```python
from build123d import *

# Parameters (mm, degrees)
SKETCH_1_R          = 103
EXTRUDE_1_DEPTH     = 3
SKETCH_2_W          = 30
SKETCH_2_H          = 42
SKETCH_2_W_2        = 24
SKETCH_2_H_2        = 32
EXTRUDE_2_DEPTH     = 25
SKETCH_3_R          = 0.5
CUT_EXTRUDE_1_DEPTH = 25
CUT_EXTRUDE_2_DEPTH = 25
SKETCH_5_R          = 103
SKETCH_5_R_2        = 100.319489632
EXTRUDE_3_DEPTH     = 50
SKETCH_6_W          = 139.713993572
SKETCH_6_H          = 16
SKETCH_6_W_2        = 184
SKETCH_6_W_3        = 75
CUT_EXTRUDE_3_DEPTH = 50
EXTRUDE_START       = -5
SKETCH_7_R          = 103
SKETCH_7_R_2        = 98
EXTRUDE_4_DEPTH     = 5
SKETCH_8_R          = 100
SKETCH_8_R_2        = 98
EXTRUDE_5_DEPTH     = 5
EXTRUDE_6_DEPTH     = 25
SKETCH_10_W         = 24
SKETCH_10_H         = 32
SKETCH_10_W_2       = 12.5
SKETCH_10_H_2       = 24
EXTRUDE_7_DEPTH     = 25
SKETCH_11_R         = 25.806975801
SKETCH_11_W         = 12.5
SKETCH_11_H         = 24
CUT_EXTRUDE_4_DEPTH = 8
SKETCH_12_W         = 12.5
SKETCH_12_H         = 24
CUT_EXTRUDE_5_DEPTH = 8
SKETCH_13_W         = 12.5
SKETCH_13_H         = 5.2
CUT_EXTRUDE_6_DEPTH = 100
SKETCH_14_R         = 103
SKETCH_14_R_2       = 98
EXTRUDE_9_DEPTH     = 50
SKETCH_15_W         = 3
SKETCH_15_H         = 9
CUT_EXTRUDE_7_DEPTH = 70


with BuildPart() as part:
    # 草图1 → 凸台-拉伸1 (new body)
    with BuildSketch(Plane(origin=(0, 0, 0), x_dir=(1, 0, 0), z_dir=(0, 1, 0))):
        with Locations(Location((0, 0, 0), (0, 0, 270))):
            Circle(SKETCH_1_R)
    extrude(amount=EXTRUDE_1_DEPTH)

    # 草图2 → 凸台-拉伸2 (add)
    with BuildSketch(Plane(origin=(0, 3, 0), x_dir=(1, 0, 0), z_dir=(0, 1, 0))):
        Rectangle(SKETCH_2_W, SKETCH_2_H)
        Rectangle(SKETCH_2_W_2, SKETCH_2_H_2, mode=Mode.SUBTRACT)
    extrude(amount=EXTRUDE_2_DEPTH)

    # 草图3 → 切除-拉伸1 (cut)
    with BuildSketch(Plane(origin=(0, 28, 0), x_dir=(1, 0, 0), z_dir=(0, 1, 0))):
        with Locations(Location((0, -18.5, 0), (0, 0, 270))):
            Circle(SKETCH_3_R)
        with Locations(Location((0, 18.5, 0), (0, 0, 270))):
            Circle(SKETCH_3_R)
    extrude(amount=-CUT_EXTRUDE_1_DEPTH, mode=Mode.SUBTRACT)

    # 草图4 → 切除-拉伸2 (cut)
    with BuildSketch(Plane(origin=(0, 3, 0), x_dir=(1, 0, 0), z_dir=(0, 1, 0))):
        Polygon((25, 0), (25, -8), (100, -8), (100, 0), (100, 8), (25, 8), align=None)
    extrude(amount=-CUT_EXTRUDE_2_DEPTH, mode=Mode.SUBTRACT)

    # 草图5 → 凸台-拉伸3 (add)
    with BuildSketch(Plane(origin=(0, 3, 0), x_dir=(1, 0, 0), z_dir=(0, 1, 0))):
        with Locations(Location((0, 0, 0), (0, 0, 270))):
            Circle(SKETCH_5_R)
        with Locations(Location((0, 0, 0), (0, 0, 4.57392126))):
            Circle(SKETCH_5_R_2, mode=Mode.SUBTRACT)
    extrude(amount=EXTRUDE_3_DEPTH)

    # 草图6 → 切除-拉伸3 (cut)
    with BuildSketch(Plane(origin=(0, 3, 0), x_dir=(1, 0, 0), z_dir=(0, 1, 0))):
        with Locations((0, -64)):
            Rectangle(SKETCH_6_W, SKETCH_6_H)
        with Locations((0, -32)):
            Rectangle(SKETCH_6_W_2, SKETCH_6_H)
        with Locations((-62.5, 0)):
            Rectangle(SKETCH_6_W_3, SKETCH_6_H)
        with Locations((0, 32)):
            Rectangle(SKETCH_6_W_2, SKETCH_6_H)
        with Locations((0, 64)):
            Rectangle(SKETCH_6_W, SKETCH_6_H)
    extrude(amount=-CUT_EXTRUDE_3_DEPTH, mode=Mode.SUBTRACT)

    # 草图7 → 凸台-拉伸4 (add)
    with BuildSketch(Plane(origin=(0, 53, 0), x_dir=(1, 0, 0), z_dir=(0, 1, 0)).offset(EXTRUDE_START)):
        with Locations(Location((0, 0, 0), (0, 0, 270))):
            Circle(SKETCH_7_R)
        with Locations(Location((0, 0, 0), (0, 0, 270))):
            Circle(SKETCH_7_R_2, mode=Mode.SUBTRACT)
    extrude(amount=EXTRUDE_4_DEPTH)

    # 草图8 → 凸台-拉伸5 (add)
    with BuildSketch(Plane(origin=(0, 53, 0), x_dir=(1, 0, 0), z_dir=(0, 1, 0))):
        with Locations(Location((0, 0, 0), (0, 0, 270))):
            Circle(SKETCH_8_R)
        with Locations(Location((0, 0, 0), (0, 0, 270))):
            Circle(SKETCH_8_R_2, mode=Mode.SUBTRACT)
    extrude(amount=EXTRUDE_5_DEPTH)

    # 草图9 → 凸台-拉伸6 (add)
    with BuildSketch(Plane(origin=(0, 28, 0), x_dir=(1, 0, 0), z_dir=(0, 1, 0))):
        with BuildLine():
            ThreePointArc((25.806975801, 0), (22.946727839, 11.808796784), (15, 21))
            Line((15, 21), (15, -21))
            ThreePointArc((15, -21), (22.946727839, -11.808796784), (25.806975801, 0))
        make_face()
        with BuildLine():
            ThreePointArc((15, 21), (0, 25.806975801), (-15, 21))
            Line((-15, 21), (15, 21))
        make_face()
        with BuildLine():
            Line((-15, -21), (-15, 21))
            ThreePointArc((-15, 21), (-25.806975801, 0), (-15, -21))
        make_face()
        with BuildLine():
            Line((15, -21), (-15, -21))
            ThreePointArc((-15, -21), (0, -25.806975801), (15, -21))
        make_face()
    extrude(amount=-EXTRUDE_6_DEPTH)

    # 草图10 → 凸台-拉伸7 (add)
    with BuildSketch(Plane(origin=(0, 28, 0), x_dir=(1, 0, 0), z_dir=(0, 1, 0))):
        Rectangle(SKETCH_10_W, SKETCH_10_H)
        Rectangle(SKETCH_10_W_2, SKETCH_10_H_2, mode=Mode.SUBTRACT)
    extrude(amount=-EXTRUDE_7_DEPTH)

    # 草图11 → 切除-拉伸4 (cut)
    with BuildSketch(Plane(origin=(0, 28, 0), x_dir=(1, 0, 0), z_dir=(0, 1, 0))):
        with Locations(Location((0, 0, 0), (0, 0, 270))):
            Circle(SKETCH_11_R)
        Rectangle(SKETCH_11_W, SKETCH_11_H, mode=Mode.SUBTRACT)
    extrude(amount=-CUT_EXTRUDE_4_DEPTH, mode=Mode.SUBTRACT)

    # 草图12 → 切除-拉伸5 (cut)
    with BuildSketch(Plane.XZ):
        Rectangle(SKETCH_12_W, SKETCH_12_H)
    extrude(amount=-CUT_EXTRUDE_5_DEPTH, mode=Mode.SUBTRACT)

    # 草图13 → 切除-拉伸6 (cut)
    with BuildSketch(Plane(origin=(0, 20, 0), x_dir=(1, 0, 0), z_dir=(0, 1, 0))):
        with Locations((0, -14.6)):
            Rectangle(SKETCH_13_W, SKETCH_13_H)
    extrude(amount=-CUT_EXTRUDE_6_DEPTH, mode=Mode.SUBTRACT)

    # 草图14 → 凸台-拉伸9 (add)
    with BuildSketch(Plane(origin=(0, 3, 0), x_dir=(1, 0, 0), z_dir=(0, 1, 0))):
        with Locations(Location((0, 0, 0), (0, 0, 270))):
            Circle(SKETCH_14_R)
        with Locations(Location((0, 0, 0), (0, 0, 270))):
            Circle(SKETCH_14_R_2, mode=Mode.SUBTRACT)
    extrude(amount=EXTRUDE_9_DEPTH)

    # 草图15 → 切除-拉伸7 (cut)
    with BuildSketch(Plane(origin=(0, 58, 0), x_dir=(1, 0, 0), z_dir=(0, 1, 0))):
        with Locations((100, 0)):
            Rectangle(SKETCH_15_W, SKETCH_15_H)
    extrude(amount=-CUT_EXTRUDE_7_DEPTH, mode=Mode.SUBTRACT)


solid = part.part
```
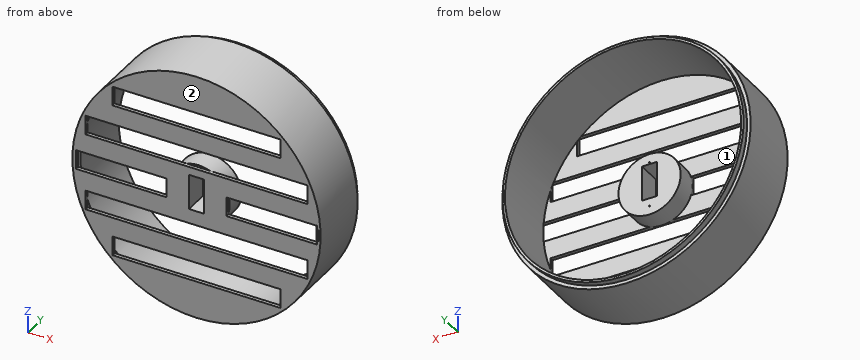
Verification items for the finished model (mm, model axes). Face numbers are marked on the shaded views. A direction names the side the tool comes from. Round coordinates to 2 decimals unless told otherwise and drop trailing zeros. Order: outer loops, then holes, each group sorted by start corner. A loop starts at its lowest first (then second) coordinate and runs counter-clockwise, first axis right, second up. Notation, with made-up numbers: (-19.75, -4.75) - (6.25, -4.75) arc R29 ccw to (6.25, 16.25) - close; hole circle Ø6 at (9, 80). An arc over 180 degrees is marked (long way). Use CSV: the item, a comma, the result in double quotes.
(1) Section check B-B on x = 63. State how many separate pieces and enclosed holes the cut face has, and give its area (3 significant figures).
Entries:
separate pieces,"6"
enclosed holes,"0"
area,"917 mm^2"
(2) Section check A-A on z = 0. Record the boundary of the cut face in (x, y), and give its area (3 significant figures).
Entries:
outline,"(-103, 0) - (-100, 0) - (-100, 3) - (-98, 3) - (-98, 58) - (-100, 58) - (-100, 53) - (-103, 53) - close; (-25.81, 3) - (-25, 3) - (-25, 0) - (-6.25, 0) - (-6.25, 20) - (-25.81, 20) - close; (6.25, 0) - (25, 0) - (25, 3) - (25.81, 3) - (25.81, 20) - (6.25, 20) - close; (98, 3) - (98.5, 3) - (98.5, 58) - (98, 58) - close; (101.5, 0) - (103, 0) - (103, 53) - (101.5, 53) - close"
area,"1,150 mm^2"
(3) Thickness scan on probe 1 along Z at (x, y) = (-1, 16); probe 2 along X at (y, z) = (46, 0); probe 3 along Z at (x, y) = (3, 45.5). Record the ranges inside material, lowest first. Write a range as from..to.
Entries:
probe 1,"-103..-97.99, -25.79..-12, 17.2..25.79, 97.99..103"
probe 2,"-103..-98, 98..98.5, 101.5..103"
probe 3,"-102.96..-97.95, 97.95..102.96"
(4) Access from +Z, -Z, +X, -X, +Y, -Y to the whole of each face (thin tool, end or side, straight path). Record for the marked faces 1 and 2.
Entries:
face 1,"+Y"
face 2,"+Z, -Z, +X, -X, -Y"
(5) Section check C-C on y = 38. Record the boundary of the cut face in (x, z).
Entries:
outline,"circle Ø206 at (0, 0); hole circle Ø196 at (0, 0); hole (98.5, -4.5) - (101.5, -4.5) - (101.5, 4.5) - (98.5, 4.5) - close"
(6) Gauge pin test, flat ends, axial feed: pin 1 Ø13 at (x, z) = (-12.5, 85.5) entering from +Y; pin 2 Ø1 at (x, z) = (-68, -70.5) entering from -Y; pin 3 Ø15.5 at (x, z) = (10, -7.5) entering from +Y. Record the tip position at first contact, or that the pin passes through.
Entries:
pin 1,"y = 3"
pin 2,"y = 3"
pin 3,"y = 20"
(7) Section check D-D on z = 64.5. Record the boundary of the cut face in (x, y).
Entries:
outline,"(-80.3, 0) - (-69.86, 0) - (-69.86, 3) - (-73.78, 3) - (-73.78, 58) - (-76.42, 58) - (-76.42, 53) - (-80.3, 53) - close; (69.86, 0) - (80.3, 0) - (80.3, 53) - (76.42, 53) - (76.42, 58) - (73.78, 58) - (73.78, 3) - (69.86, 3) - close"
